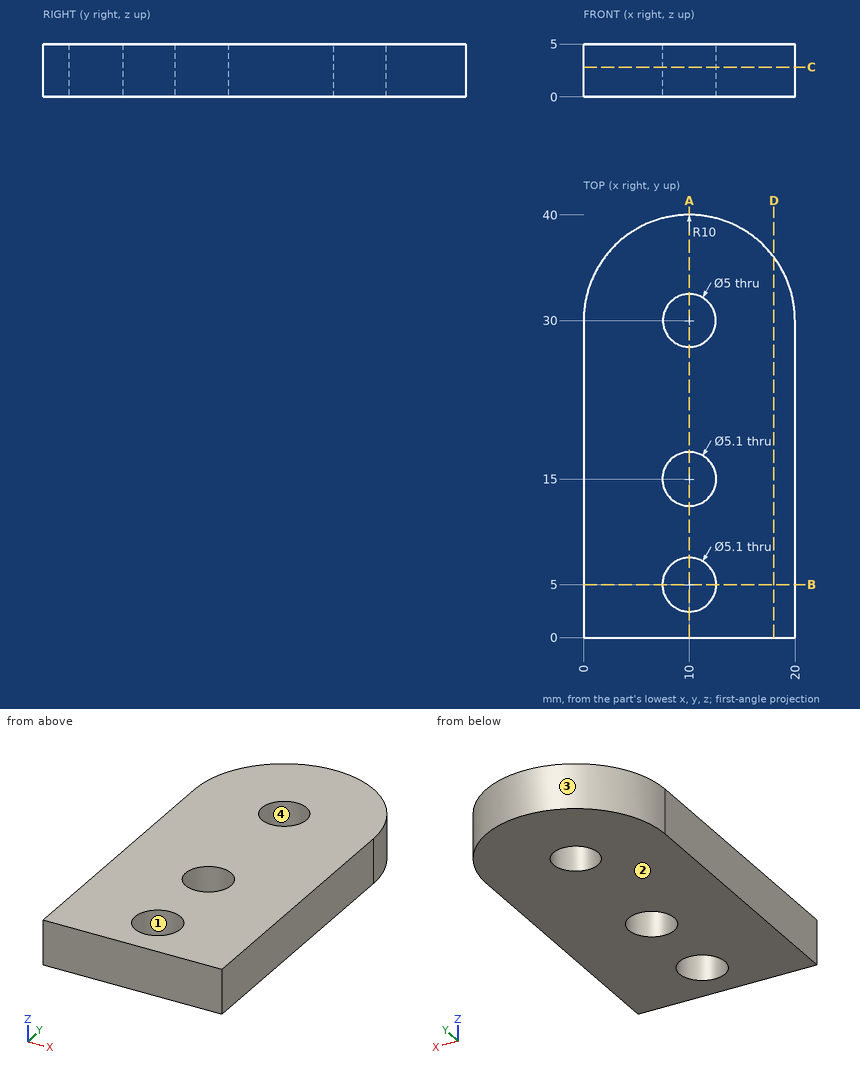
Check sheet for the drawn part. Datum: minimum x, y, z corner. Units: mm. Round coordinates to 2 decimals unless told otherwise and drop trailing zeros. Order: outer loops, then holes, each group sorted by start corner. A loop starts at its lowest first (then second) coordinate and runs counter-clockwise, first axis right, second up.
(1) Draft check along Y on the marked faces 1, 2, 3 and 4. Enter one of: pulls with the +Y half, pulls with the -Y half, needs draft (parallel to the pull), parting line crosses it, or undercut.
(2) Scan lines: probe 1 along Y at (x, z) = (10, 3.8); probe 2 along Y at (x, z) = (7.75, 0.4); probe 3 along Y at (x, z) = (16.25, 3.1). Record each from-to range of solid material in increasing order.
(3) Cross-section at B-B, the plane y = 5. Enter the section's corners in (x, z), and give its area (3 significant figures).
(4) Go/stop test with flat-tipped pins: P1, Ø3, axis at x = 10, y = 5, coming from the +Z side; P2, Ø1.5, axis at y = 32.5, z = 1, coming from the -X side. Record where each tip stops, or that it passes through.
(5) Cross-section at A-A, the plane x = 10. Enter the section's corners in (y, z).
(6) Cross-section at C-C, the plane z = 2.8. Enter the section's corners in (x, y), and give its area (3 significant figures).
(7) Cross-section at D-D, the plane x = 18. Enter the section's corners in (y, z).
Check sheet entries:
1. face 1: undercut
1. face 2: needs draft
1. face 3: pulls with the +Y half
1. face 4: undercut
2. probe 1: y = 0 to 2.45, 7.55 to 12.45, 17.55 to 27.5, 32.5 to 40
2. probe 2: y = 0 to 3.8, 6.2 to 13.8, 16.2 to 28.91, 31.09 to 39.74
2. probe 3: y = 0 to 37.81
3. outline: (0, 0) - (7.45, 0) - (7.45, 5) - (0, 5) - close; (12.55, 0) - (20, 0) - (20, 5) - (12.55, 5) - close
3. area: 74.5 mm2
4. P1: passes through
4. P2: stops at x = 0.15
5. outline: (0, 0) - (2.45, 0) - (2.45, 5) - (0, 5) - close; (7.55, 0) - (12.45, 0) - (12.45, 5) - (7.55, 5) - close; (17.55, 0) - (27.5, 0) - (27.5, 5) - (17.55, 5) - close; (32.5, 0) - (40, 0) - (40, 5) - (32.5, 5) - close
6. outline: (0, 0) - (20, 0) - (20, 30) arc R10 ccw to (0, 30) - close; hole circle Ø5.1 at (10, 5); hole circle Ø5.1 at (10, 15); hole circle Ø5 at (10, 30)
6. area: 697 mm2
7. outline: (0, 0) - (36, 0) - (36, 5) - (0, 5) - close
